Geometry: see drawing. Coordinates: mm, zero at the bounding-box minimum. A direction names the side the tool comes from. Round coordinates to 2 decimals unless told otherwise and drop trailing zeros. Loops run counter-clockwise (first coordinate to the right, second up) from the corner with the lowest first, then second, coordinate; pieces in that order, holes last. Notation, with made-up numbers: (74, 59) -> (114, 59) arc R9 ccw to (114, 69) -> close; hole circle Ø8 at (81.25, -36). An arc over 180 degrees is marked (long way). Answer in a Markdown table with one row per item.
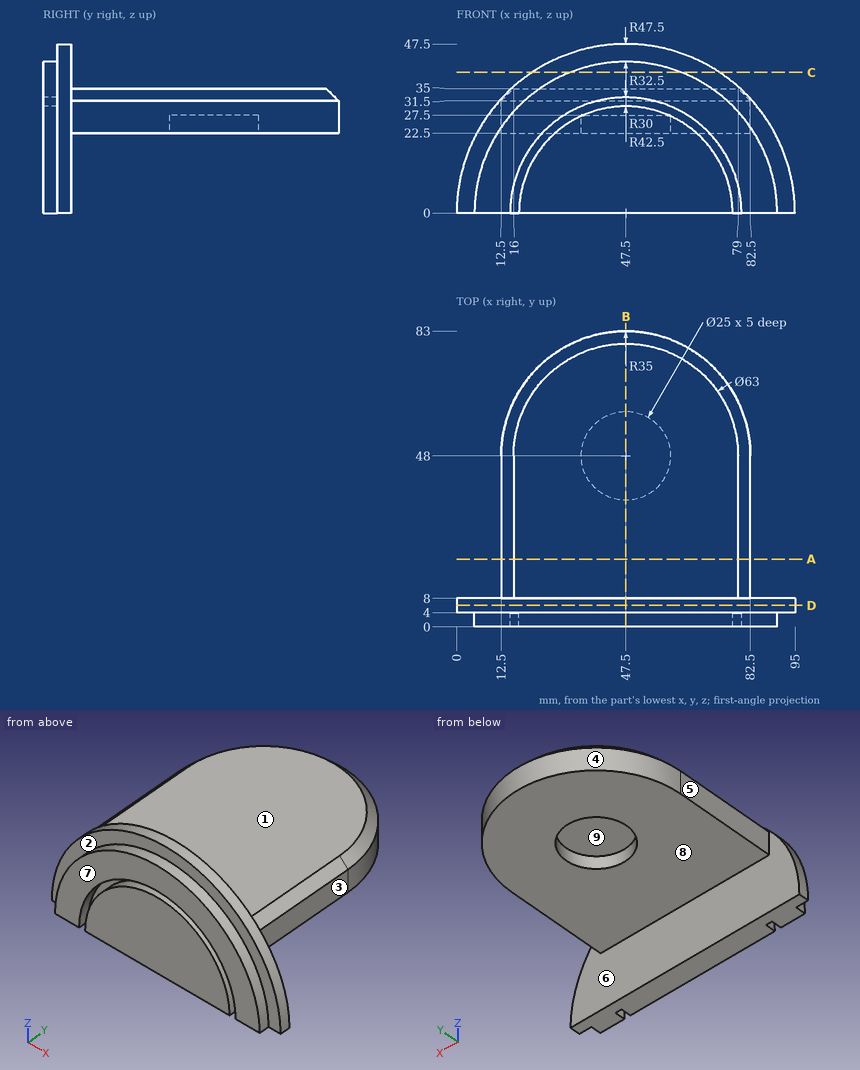
Item 1: Section query B-B, the plane x = 47.5. Output: boundary loops of the cut face in (y, z).
Ans:
| item | result |
|---|---|
| outline | (0, 0) -> (8, 0) -> (8, 22.5) -> (35.5, 22.5) -> (35.5, 27.5) -> (60.5, 27.5) -> (60.5, 22.5) -> (83, 22.5) -> (83, 31.5) -> (79.5, 35) -> (8, 35) -> (8, 47.5) -> (4, 47.5) -> (4, 42.5) -> (0, 42.5) -> (0, 32.5) -> (4, 32.5) -> (4, 30) -> (0, 30) -> close |
Item 2: First-contact query: P1, Ø2, axis at x = 49.5, z = 24, coming from the +Y side; P2, Ø6, axis at x = 52.5, y = 54, coming from the +Z side; P3, Ø12.5, axis at x = 44.5, y = 51, coming from the -Z side. Flat tips, straight axial feed; report the tip coordinate or a pass-through.
Ans:
| item | result |
|---|---|
| P1 | y = 82.99 |
| P2 | z = 35 |
| P3 | z = 27.5 |
Item 3: Mould query, pull axis Y, two halves, no side actions, for the marked faces 6, 7, 8 and 9. Classes: released by +Y, released by -Y, zero draft, split by the parting line, or undercut.
Ans:
| item | result |
|---|---|
| face 6 | released by +Y |
| face 7 | released by -Y |
| face 8 | zero draft |
| face 9 | undercut |
Item 4: Section query C-C, the plane z = 39.5. Output: boundary loops of the cut face in (x, y), and give its area (3 significant figures).
Ans:
| item | result |
|---|---|
| outline | (21.12, 4) -> (31.82, 4) -> (31.82, 0) -> (63.18, 0) -> (63.18, 4) -> (73.88, 4) -> (73.88, 8) -> (21.12, 8) -> close |
| area | 337 mm2 |
Item 5: Section query A-A, the plane y = 19. Output: boundary loops of the cut face in (x, z), and give its area (3 significant figures).
Ans:
| item | result |
|---|---|
| outline | (12.5, 22.5) -> (82.5, 22.5) -> (82.5, 31.5) -> (79, 35) -> (16, 35) -> (12.5, 31.5) -> close |
| area | 863 mm2 |
Item 6: Ray query, L1, parallel to Y at x = 47, z = 25; L2, parallel to Z at x = 52, y = 43.5; L3, parallel to Z at x = 73, y = 10.5. Return the intervals inside material, ascending.
Ans:
| item | result |
|---|---|
| L1 | 0 to 35.51, 60.49 to 83 |
| L2 | 27.5 to 35 |
| L3 | 22.5 to 35 |
Item 7: Section query D-D, the plane y = 6. Output: boundary loops of the cut face in (x, z).
Ans:
| item | result |
|---|---|
| outline | (0, 0) -> (95, 0) arc R47.5 ccw to start |
Item 8: Set-up query: the marked faces 1, 2, 3, 4 and 5. Return all of +Z, -Z, +X, -X, +Y, -Y with unobstructed straight access to the full face (end or side cutting, diameter ignored); none if empty.
Ans:
| item | result |
|---|---|
| face 1 | +Z, +X, -X, +Y |
| face 2 | +Z, -Y |
| face 3 | +Z, -Z, +X, +Y |
| face 4 | +Z, -Z, +Y |
| face 5 | +Z, -Z, -X, +Y |
